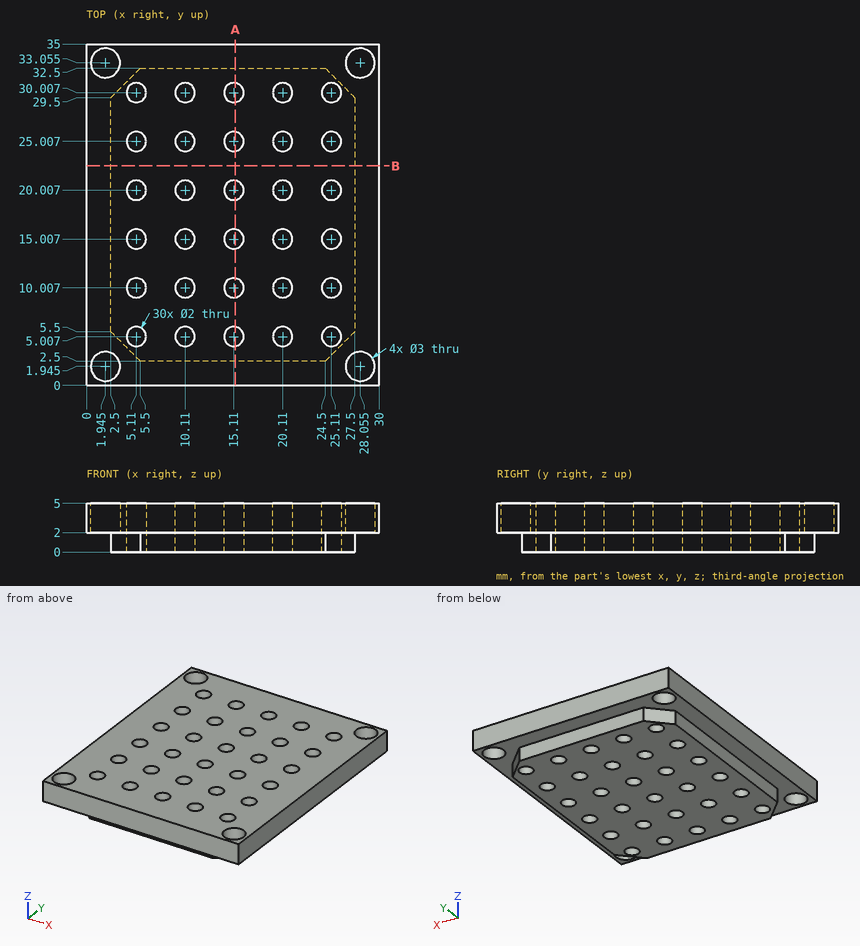
Geometry: see drawing. Coordinates: mm, zero at the bounding-box minimum. Give positions to 0.01 mm unless a question says otherwise; leave off trailing zeros. Write each loop counter-clockwise with the first axis right and the second up, starting at its lowest first coordinate (ties: lowest second). Pieces come first, ordered by that corner, then holes. Notation, with made-up numbers: M -15.5,14 L 27.5,14 A24 ccw 27.5,25 Z; hole C -4,12.5 d4. An arc over 180 degrees is marked long. Return JSON: item names as keys, results as strings. Group by question number.
1) First-contact query: pin 1 Ø1.6 at (y, z) = (14.5, 1) entering from -X; pin 2 Ø1.2 at (x, y) = (15.11, 25.01) entering from -Z; pin 3 Ø2 at (x, z) = (19, 0.5) entering from -Y. Flat tips, straight axial feed; report the tip coordinate or a pass-through.
2) Cut plane B-B, the plane y = 22.5. Output: boundary loops of the cut face in (x, z), then the cut area to 3 significant figures.
3) Cut plane A-A, the plane x = 15.25. Give the number of separate pieces and of enclosed holes in the cut face.
4) Ray query, L1, parallel to Y at x = 3.25, z = 4 (1 decimal); L2, parallel to X at y = 20.5, z = 1.45; L3, parallel to Y at x = 2.5, z = 2.65. Return the intervals inside material, ascending.
Data:
{
 "1": {"pin 1": "stops at x = 2.5", "pin 2": "passes through", "pin 3": "stops at y = 2.5"},
 "2": {"outline": "M 0,2 L 2.5,2 L 2.5,0 L 27.5,0 L 27.5,2 L 30,2 L 30,5 L 0,5 Z", "area": "140 mm²"},
 "3": {"separate pieces": "7", "enclosed holes": "0"},
 "4": {"L1": "y = 0 to 1.2, 2.7 to 32.3, 33.8 to 35", "L2": "x = 2.5 to 4.24, 5.98 to 9.24, 10.98 to 14.24, 15.98 to 19.24, 20.98 to 24.24, 25.98 to 27.5", "L3": "y = 0 to 0.55, 3.34 to 31.66, 34.45 to 35"}
}
